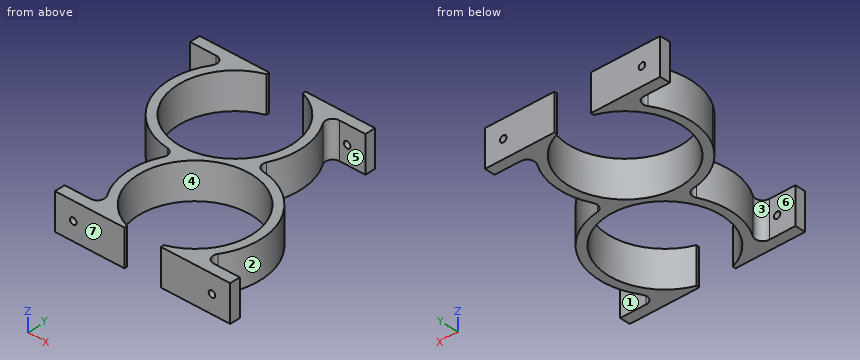
```python
from build123d import *

# Parameters (mm, degrees)
F1_DEPTH       = 12.7
F6_D           = 2.2606
F6_DEPTH       = 12.7
F6_TIP         = 0.6791527577
F6_ON_F5_D     = 2.2606
F6_ON_F5_DEPTH = 12.7
F6_ON_F5_TIP   = 0.6791527577
F6_ON_F2_D     = 2.2606
F6_ON_F2_DEPTH = 12.7
F6_ON_F2_TIP   = 0.6791527577
F6_ON_F3_D     = 2.2606
F6_ON_F3_DEPTH = 12.7
F6_ON_F3_TIP   = 0.6791527577


with BuildPart() as f1:
    # F0 (on Top) → F1 (new body)
    with BuildSketch(Plane.XY):
        with BuildLine():
            Line((0.2285717149, -38.1), (19.2785717149, -38.1))
            Line((19.2785717149, -38.1), (19.2785717149, -34.4883422186))
            Line((19.2785717149, -34.4883422186), (10.2378985351, -34.4883422186))
            ThreePointArc((10.2378985351, -34.4883422186), (8.0106438434, -33.1693813409), (8.0965086816, -30.5823079967))
            ThreePointArc((8.0965086816, -30.5823079967), (9.4676308494, -8.4686260202), (-8.553227146, 4.4210436293))
            ThreePointArc((-8.553227146, 4.4210436293), (-10.495209535, 5.7345115019), (-10.534427146, 8.0786436293))
            ThreePointArc((-10.534427146, 8.0786436293), (-8.1594188782, 19.4861168414), (-11.7154913184, 30.5823079967))
            ThreePointArc((-11.7154913184, 30.5823079967), (-11.8013561566, 33.1693813409), (-9.5741014649, 34.4883422186))
            Line((-9.5741014649, 34.4883422186), (-0.5334282851, 34.4883422186))
            Line((-0.5334282851, 34.4883422186), (-0.5334282851, 38.1))
            Line((-0.5334282851, 38.1), (-24.638, 38.1))
            Line((-24.638, 38.1), (-24.638, 37.0548016455))
            ThreePointArc((-24.638, 37.0548016455), (-30.988, -1.524), (-37.338, 37.0548016455))
            Line((-37.338, 37.0548016455), (-37.338, 38.1))
            Line((-37.338, 38.1), (-61.4425717149, 38.1))
            Line((-61.4425717149, 38.1), (-61.4425717149, 34.4883422186))
            Line((-61.4425717149, 34.4883422186), (-52.4018985351, 34.4883422186))
            ThreePointArc((-52.4018985351, 34.4883422186), (-50.1746438434, 33.1693813409), (-50.2605086816, 30.5823079967))
            ThreePointArc((-50.2605086816, 30.5823079967), (-53.8420790586, 18.8082599192), (-50.8, 6.8834282851))
            ThreePointArc((-50.8, 6.8834282851), (-43.5489525741, -0.8117924185), (-33.610772854, -4.4210436293))
            ThreePointArc((-33.610772854, -4.4210436293), (-31.668790465, -5.7345115019), (-31.629572854, -8.0786436293))
            ThreePointArc((-31.629572854, -8.0786436293), (-34.0045811218, -19.4861168414), (-30.4485086816, -30.5823079967))
            ThreePointArc((-30.4485086816, -30.5823079967), (-30.3626438434, -33.1693813409), (-32.5898985351, -34.4883422186))
            Line((-32.5898985351, -34.4883422186), (-41.6305717149, -34.4883422186))
            Line((-41.6305717149, -34.4883422186), (-41.6305717149, -38.1))
            Line((-41.6305717149, -38.1), (-22.5805717149, -38.1))
            Line((-22.5805717149, -38.1), (-17.526, -38.1))
            Line((-17.526, -38.1), (-17.526, -37.0548016455))
            ThreePointArc((-17.526, -37.0548016455), (-11.176, 1.524), (-4.826, -37.0548016455))
            Line((-4.826, -37.0548016455), (-4.826, -38.1))
            Line((-4.826, -38.1), (0.2285717149, -38.1))
        make_face()
    extrude(amount=F1_DEPTH)

    # F6
    with Locations(Plane(origin=(0, 38.1, 0), x_dir=(-1, 0, 0), z_dir=(0, 1, 0))):
        with Locations((55.0925717149, 6.35)):
            Hole(F6_D / 2, depth=F6_DEPTH)
            with Locations((0, 0, -(F6_DEPTH + F6_TIP / 2))):  # 118° drill point
                Cone(0, F6_D / 2, F6_TIP, mode=Mode.SUBTRACT)

    # F6 on F5
    with Locations(Plane(origin=(0, 38.1, 0), x_dir=(-1, 0, 0), z_dir=(0, 1, 0))):
        with Locations((6.8834282851, 6.35)):
            Hole(F6_ON_F5_D / 2, depth=F6_ON_F5_DEPTH)
            with Locations((0, 0, -(F6_ON_F5_DEPTH + F6_ON_F5_TIP / 2))):  # 118° drill point
                Cone(0, F6_ON_F5_D / 2, F6_ON_F5_TIP, mode=Mode.SUBTRACT)

    # F6 on F2
    with Locations(Plane.XZ.offset(38.1)):
        with Locations((-35.2805717149, 6.35)):
            Hole(F6_ON_F2_D / 2, depth=F6_ON_F2_DEPTH)
            with Locations((0, 0, -(F6_ON_F2_DEPTH + F6_ON_F2_TIP / 2))):  # 118° drill point
                Cone(0, F6_ON_F2_D / 2, F6_ON_F2_TIP, mode=Mode.SUBTRACT)

    # F6 on F3
    with Locations(Plane.XZ.offset(38.1)):
        with Locations((12.9285717149, 6.35)):
            Hole(F6_ON_F3_D / 2, depth=F6_ON_F3_DEPTH)
            with Locations((0, 0, -(F6_ON_F3_DEPTH + F6_ON_F3_TIP / 2))):  # 118° drill point
                Cone(0, F6_ON_F3_D / 2, F6_ON_F3_TIP, mode=Mode.SUBTRACT)


solid = f1.part
```
Check sheet for the modelled part. Datum: model origin and axes. Units: mm. Face numbers are marked on the shaded views. A direction names the side the tool comes from. Round coordinates to 2 decimals unless told otherwise and drop trailing zeros. Write each loop counter-clockwise with the first axis right and the second up, starting at its lowest first coordinate (ties: lowest second). Pieces come first, ordered by that corner, then holes. Notation, with made-up numbers: M -31,-24.5 L 9,-24.5 A19 cw 9,4.5 Z; hole C 86.5,60.25 d5. An arc over 180 degrees is marked long. Write item = value, one per line. Start each with the question number.
1. Gauge pin test, flat ends, axial feed: pin 1 (1.4 mm diameter, centred on x = -35.28, z = 6.35, fed in from +Y); pin 2 (0.8 mm diameter, centred on y = 37.5, z = 4, fed in from +X); pin 3 (7 mm diameter, centred on x = -59, z = 9.5, fed in from -Y). Record the tip position at first contact, or that the pin passes through.
2. Release check for a two-part mould opening along X. For the marked faces 1, 2, 3 and 4 record: pulls with the +X half, pulls with the -X half, needs draft (parallel to the pull), parting line crosses it, or undercut.
3. Section check D-D, the plane z = 6.35. State how many separate pieces and enclosed holes the cut face has, then the cut area to 3 significant figures.
4. Section check C-C, the plane z = 10.5. Record the cut outline in (x, y), then the cut area to 3 significant figures.
5. Section check B-B, the plane x = -46.5. Record the cut outline in (y, z), then the cut area to 3 significant figures.
6. Scan lines: line 1 (X direction, y = -18.5, z = 10.75); line 2 (Y direction, x = -40, z = 12); line 3 (Y direction, x = -21, z = 1.25). Record each from-to range of solid material in increasing order. Write a range as [from, to].
7. Section check A-A, the plane y = -29. Record the cut outline in (x, z).
8. Tool access check on the marked faces 5, 6 and 7. Record the directions out of +Z, -Z, +X, -X, +Y, -Y that give a thin tool (end or side, any length) a straight path to the whole face; none if there is none.
Results found:
q1.pin_1 = -0.88
q1.pin_2 = -0.53
q1.pin_3 = 34.49
q2.face_1 = needs draft
q2.face_2 = pulls with the +X half
q2.face_3 = pulls with the -X half
q2.face_4 = undercut
q3.separate_pieces = 5
q3.enclosed_holes = 0
q3.area = 898 mm^2
q4.outline = M -61.44,34.49 L -52.4,34.49 A2.54 cw -50.26,30.58 A22.86 ccw -33.61,-4.42 A2.54 cw -31.63,-8.08 A22.86 ccw -30.45,-30.58 A2.54 cw -32.59,-34.49 L -41.63,-34.49 L -41.63,-38.1 L -17.53,-38.1 L -17.53,-37.05 A19.81 cw long -4.83,-37.05 L -4.83,-38.1 L 19.28,-38.1 L 19.28,-34.49 L 10.24,-34.49 A2.54 cw 8.1,-30.58 A22.86 ccw -8.55,4.42 A2.54 cw -10.53,8.08 A22.86 ccw -11.72,30.58 A2.54 cw -9.57,34.49 L -0.53,34.49 L -0.53,38.1 L -24.64,38.1 L -24.64,37.05 A19.81 cw long -37.34,37.05 L -37.34,38.1 L -61.44,38.1 Z
q4.area = 930 mm^2
q5.outline = M 1.5,0 L 5.96,0 L 5.96,12.7 L 1.5,12.7 Z; M 30.61,0 L 38.1,0 L 38.1,12.7 L 30.61,12.7 Z
q5.area = 152 mm^2
q6.line_1 = [-34.04, -30.99], [8.63, 11.68]
q6.line_2 = [-38.1, -34.49], [-2.72, 0.64], [35.93, 38.1]
q6.line_3 = [-38.1, -35.49], [-1.08, 1.18], [35.4, 38.1]
q7.outline = M -31.37,0 L -27.84,0 L -27.84,12.7 L -31.37,12.7 Z; M 5.49,0 L 9.02,0 L 9.02,12.7 L 5.49,12.7 Z
q8.face_5 = +Z, -Z, +X
q8.face_6 = +Z, -Z, -X
q8.face_7 = +Z, -Z, +X, -X, -Y
